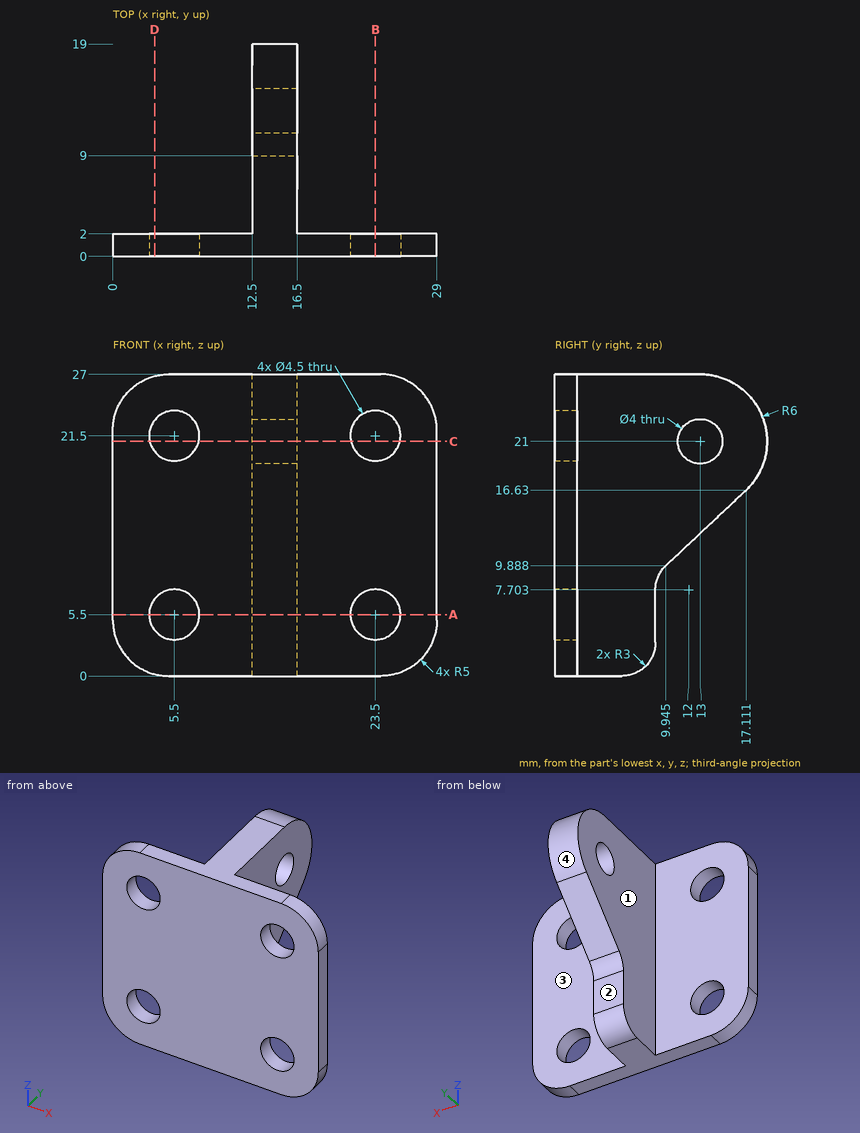
Design review of the part shown in the three views and the two pictorial views. Dimensions are in mm from the part's minimum x, y and z. A direction names the side the tool comes from. Round coordinates to 2 decimals unless told otherwise and drop trailing zeros. Write each loop counter-clockwise with the first axis right and the second up, starting at its lowest first coordinate (ties: lowest second). Pieces come first, ordered by that corner, then holes.
Item 1: Consider section D-D on x = 3.75. Give the boundary of the cut face in (y, z) (1 decimal).
Item 2: Consider section B-B on x = 23.5. Give the boundary of the cut face in (y, z), and give its area (3 significant figures).
Item 3: Consider section C-C on z = 21. Give the boundary of the cut face in (x, y).
Item 4: For pin 1 Ø10 at (y, z) = (9, 10.5) entering from -X; pin 2 Ø6 at (x, z) = (4, 7) entering from +Y; pin 3 Ø1 at (x, z) = (25.5, 21.5) entering from -Y; pin 4 Ø4.5 at (x, z) = (13.5, 5) entering from +Y, all flat-tipped, find the tip position at first contact; note any pin that passes through.
Item 5: Wall thickness on L1, parallel to X at y = 0.45, z = 21.5; L2, parallel to Y at x = 14.5, z = 21; L3, parallel to X at y = 15.5, z = 18: over which ranges is each line inside the solid? List them lowest first.
Item 6: Consider section A-A on z = 5.5. Give the boundary of the cut face in (x, y).
Item 7: For the marked faces 1, 2, 3 and 4, list the 3-axis set-ups (+Z, -Z, +X, -X, +Y, -Y) from which the entire face can be reached by the end or side of a thin tool; tool diameter is ignored.
Check values:
1. outline: (0, 0.2) - (2, 0.2) - (2, 4.1) - (0, 4.1) - close; (0, 6.9) - (2, 6.9) - (2, 20.1) - (0, 20.1) - close; (0, 22.9) - (2, 22.9) - (2, 26.8) - (0, 26.8) - close
2. outline: (0, 0) - (2, 0) - (2, 3.25) - (0, 3.25) - close; (0, 7.75) - (2, 7.75) - (2, 19.25) - (0, 19.25) - close; (0, 23.75) - (2, 23.75) - (2, 27) - (0, 27) - close
2. area: 36.0 mm2
3. outline: (0, 0) - (3.31, 0) - (3.31, 2) - (0, 2) - close; (7.69, 0) - (21.31, 0) - (21.31, 2) - (16.5, 2) - (16.5, 11) - (12.5, 11) - (12.5, 2) - (7.69, 2) - close; (12.5, 15) - (16.5, 15) - (16.5, 19) - (12.5, 19) - close; (25.69, 0) - (29, 0) - (29, 2) - (25.69, 2) - close
4. pin 1: stops at x = 12.5
4. pin 2: stops at y = 2
4. pin 3: stops at y = 0
4. pin 4: stops at y = 9
5. L1: x = 0 to 3.25, 7.75 to 21.25, 25.75 to 29
5. L2: y = 0 to 11, 15 to 19
5. L3: x = 12.5 to 16.5
6. outline: (0, 0) - (3.25, 0) - (3.25, 2) - (0, 2) - close; (7.75, 0) - (21.25, 0) - (21.25, 2) - (16.5, 2) - (16.5, 9) - (12.5, 9) - (12.5, 2) - (7.75, 2) - close; (25.75, 0) - (29, 0) - (29, 2) - (25.75, 2) - close
7. face 1: +Z, -Z, -X, +Y
7. face 2: -Z, +X, -X, +Y
7. face 3: +Z, -Z, +X, +Y
7. face 4: +X, -X, +Y
